Build history of the part. All positions in model axes, mm. Give positions to 0.01 mm unless a question says otherwise; leave off trailing zeros. Write each loop counter-clockwise with the first axis right and the second up, starting at its lowest first coordinate (ties: lowest second). Pieces come first, ordered by that corner, then holes. Notation, with made-up numbers: M 88.5,37.25 L 126.5,37.25 A15 ccw 126.5,54.25 Z; hole C -18,45.5 d7. An arc over 180 degrees is marked long. One line per item, written item: value. Start each with the question number.
from build123d import *

# Parameters (mm, degrees)
SKETCH1_W                  = 1130
SKETCH1_H                  = 450
BOSS_EXTRUDE1_DEPTH        = 10
SKETCH2_W                  = 65
SKETCH2_H                  = 65
CUT_EXTRUDE1_DEPTH         = 11
SKETCH3_W                  = 123
SKETCH3_H                  = 125
CUT_EXTRUDE2_DEPTH         = 11
F_13_0_13_DIAMETER_HOLE1_D = 13


with BuildPart() as part:
    # Sketch1 → Boss-Extrude1 (new body)
    with BuildSketch(Plane.XY):
        with Locations((0, -25)):
            Rectangle(SKETCH1_W, SKETCH1_H)
    extrude(amount=BOSS_EXTRUDE1_DEPTH)

    # Sketch2 → Cut-Extrude1 (cut, through all)
    with BuildSketch(Plane.XY.offset(10)):
        with Locations((-532.5, 167.5)):
            Rectangle(SKETCH2_W, SKETCH2_H)
    cut_extrude1 = extrude(amount=-CUT_EXTRUDE1_DEPTH, mode=Mode.SUBTRACT)

    # Mirror1: Cut-Extrude1 across plane
    add(cut_extrude1.mirror(Plane(origin=(0, 0, 0), x_dir=(0, 0, 1), z_dir=(1, 0, 0))), mode=Mode.SUBTRACT)

    # Sketch3 → Cut-Extrude2 (cut, through all)
    with BuildSketch(Plane.XY.offset(10)):
        with Locations((110, 137.5)):
            Rectangle(SKETCH3_W, SKETCH3_H)
    extrude(amount=-CUT_EXTRUDE2_DEPTH, mode=Mode.SUBTRACT)

    # Ø13.0 (13) Diameter Hole1 (through all)
    with Locations(Plane.XY.offset(10)):
        with Locations((-365, 120), (-185, 120), (-185, -80), (-365, -80)):
            Hole(F_13_0_13_DIAMETER_HOLE1_D / 2)


solid = part.part
1) Band-saw the part on B-B (x = 126.5). List the corners of the cut face in (y, z), then the cut area to 3 significant figures.
2) Band-saw the part on A-A (z = 2.25). List the corners of the cut face in (x, y), then the cut area to 3 significant figures.
3) Drop a flat-ended pin along its axis: P1, Ø5, axis at y = 147.5, z = 6.5, coming from the +X side. Give the stop position or say it passes through.
4) Probe line 1 along Y through (x, z) = (-185, 6.5); line 2 along X through (y, z) = (85.5, 2.75); line 3 along X through (y, z) = (136, 1.5). List the from-to ranges inside material, lowest first. Write a range as from..to.
Model answer:
1. outline: M -250,0 L 75,0 L 75,10 L -250,10 Z
1. area: 3,250 mm²
2. outline: M -565,-250 L 565,-250 L 565,135 L 500,135 L 500,200 L 171.5,200 L 171.5,75 L 48.5,75 L 48.5,200 L -500,200 L -500,135 L -565,135 Z; hole C -365,-80 d13; hole C -365,120 d13; hole C -185,-80 d13; hole C -185,120 d13
2. area: 484,000 mm²
3. P1: stops at x = 500
4. line 1: y = -250..-86.5, -73.5..113.5, 126.5..200
4. line 2: x = -565..48.5, 171.5..565
4. line 3: x = -500..48.5, 171.5..500
